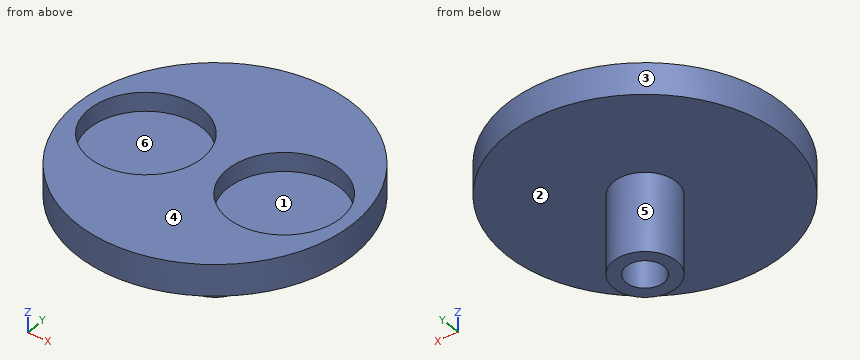
from build123d import *

# Parameters (mm, degrees)
F1_R     = 5
F1_R_2   = 3
F3_DEPTH = 12.5
F5_R     = 22
F6_DEPTH = 5
F7_R     = 9
F8_DEPTH = 3


with BuildPart() as f3:
    # F1 (on Top) → F3 (new body)
    with BuildSketch(Plane.XY):
        Circle(F1_R)
        Circle(F1_R_2, mode=Mode.SUBTRACT)
    extrude(amount=-F3_DEPTH)

    # F5 (on Top) → F6 (join)
    with BuildSketch(Plane.XY):
        Circle(F5_R)
    extrude(amount=F6_DEPTH)

    # F7 (on face) → F8 (cut)
    with BuildSketch(Plane.XY.offset(5)):
        with Locations((11, 0)):
            Circle(F7_R)
        with Locations((-11, 0)):
            Circle(F7_R)
    extrude(amount=-F8_DEPTH, mode=Mode.SUBTRACT)


solid = f3.part
Work out the finished part from the listing and answer in its coordinate system (mm). Face numbers are marked on the shaded views. A direction names the side the tool comes from. Coordinates: 2 decimals unless noted, no trailing zeros. Write each loop counter-clockwise with the first axis right and the second up, starting at its lowest first coordinate (ties: lowest second). Pieces come first, ordered by that corner, then holes.
1. For the marked faces 4, 5 and 6, determine the directions among +Z, -Z, +X, -X, +Y, -Y from which every point of the face is accessible in a straight line to the end or side of a thin tool.
Results list:
face 4: +Z, +X, -X, +Y, -Y
face 5: -Z
face 6: +Z
2. The part is cut by section B-B, the plane x = 6. Write down the section's boundary in (y, z), and give its area (3 significant figures).
Results list:
outline: (-21.17, 0) - (21.17, 0) - (21.17, 5) - (7.48, 5) - (7.48, 2) - (-7.48, 2) - (-7.48, 5) - (-21.17, 5) - close
area: 167 mm2
3. The part is cut by section C-C, the plane z = -10.5. Write down the section's boundary in (x, y), and give its area (3 significant figures).
Results list:
outline: circle Ø10 at (0, 0); hole circle Ø6 at (0, 0)
area: 50.3 mm2
4. For a pull along X with two mould halves and no side action, classify the marked faces 1, 2 and 3 as +X half, -X half, draft (parallel to the pull), parting line (faces both ways), or undercut.
Results list:
face 1: undercut
face 2: draft
face 3: parting line
5. The part is cut by section A-A, the plane y = 0. Write down the section's boundary in (x, z).
Results list:
outline: (-22, 0) - (-5, 0) - (-5, -12.5) - (-3, -12.5) - (-3, 0) - (3, 0) - (3, -12.5) - (5, -12.5) - (5, 0) - (22, 0) - (22, 5) - (20, 5) - (20, 2) - (2, 2) - (2, 5) - (-2, 5) - (-2, 2) - (-20, 2) - (-20, 5) - (-22, 5) - close
6. Consider line 1 along Z through (x, y) = (-9.5, 17); line 2 along Y through (x, z) = (4, -6.25); line 3 along Y through (x, z) = (0, -9). Determine where each line is inside the solid, lowest interval first.
Results list:
line 1: z = 0 to 5
line 2: y = -3 to 3
line 3: y = -5 to -3, 3 to 5
7. The part is cut by section D-D, the plane x = 0. Write down the section's boundary in (y, z), and give its area (3 significant figures).
Results list:
outline: (-22, 0) - (-5, 0) - (-5, -12.5) - (-3, -12.5) - (-3, 0) - (3, 0) - (3, -12.5) - (5, -12.5) - (5, 0) - (22, 0) - (22, 5) - (-22, 5) - close
area: 270 mm2
8. Flat-ended cylindrical pins translate along their axes: pin 1 (20.5 mm diameter, centred on x = 11, y = 0, fed in from +Z); pin 2 (16 mm diameter, centred on x = -11, y = 0, fed in from +Z); pin 3 (4 mm diameter, centred on y = -10.5, z = -0.5, fed in from +X); pin 4 (1 mm diameter, centred on x = -4, z = -3.5, fed in from -Y). Find the tip coordinate at first contact, or state that the pin passes through.
Results list:
pin 1: stops at z = 5
pin 2: stops at z = 2
pin 3: stops at x = 20.26
pin 4: stops at y = -3.57
